Part model, mm, in its own coordinate system. Give positions to 0.01 mm unless a question says otherwise; leave off trailing zeros. Loops run counter-clockwise (first coordinate to the right, second up) from the corner with the lowest first, then second, coordinate; pieces in that order, holes last. Notation, with made-up numbers: M 74,55 L 103,55 A23 cw 103,69 Z; hole C 33,88.25 d4. An arc over 180 degrees is marked long. Put each result on its own line as item: value. Start each with the question number.
```python
from build123d import *

# Parameters (mm, degrees)
SKETCH1_W           = 271.5
SKETCH1_H           = 84
SKETCH1_R           = 1.5
BOSS_EXTRUDE1_DEPTH = 2
SKETCH2_R           = 1.5
SKETCH2_R_2         = 7.5
CUT_EXTRUDE1_DEPTH  = 10


with BuildPart() as part:
    # Sketch1 → Boss-Extrude1 (new body)
    with BuildSketch(Plane(origin=(0, 0, 0), x_dir=(1, 0, 0), z_dir=(0, 1, 0))):
        with Locations((135.75, 42)):
            Rectangle(SKETCH1_W, SKETCH1_H)
        with Locations(Location((4, 5.75, 0), (0, 0, 270))):
            Circle(SKETCH1_R, mode=Mode.SUBTRACT)
        with Locations(Location((4, 78.25, 0), (0, 0, 270))):
            Circle(SKETCH1_R, mode=Mode.SUBTRACT)
        with Locations(Location((267.5, 5.75, 0), (0, 0, 270))):
            Circle(SKETCH1_R, mode=Mode.SUBTRACT)
        with Locations(Location((267.5, 78.25, 0), (0, 0, 270))):
            Circle(SKETCH1_R, mode=Mode.SUBTRACT)
    extrude(amount=BOSS_EXTRUDE1_DEPTH)

    # Sketch2 → Cut-Extrude1 (cut)
    with BuildSketch(Plane(origin=(0, 2, 0), x_dir=(1, 0, 0), z_dir=(0, 1, 0))):
        with Locations(Location((15, 5.5, 0), (0, 0, 270))):
            Circle(SKETCH2_R)
        with Locations(Location((15, 40.5, 0), (0, 0, 270))):
            Circle(SKETCH2_R)
        with Locations(Location((15, 23, 0), (0, 0, 270))):
            Circle(SKETCH2_R_2)
        with Locations(Location((256.5, 23, 0), (0, 0, 90))):
            Circle(SKETCH2_R_2)
        with Locations(Location((256.5, 40.5, 0), (0, 0, 90))):
            Circle(SKETCH2_R)
        with Locations(Location((256.5, 5.5, 0), (0, 0, 90))):
            Circle(SKETCH2_R)
    extrude(amount=-CUT_EXTRUDE1_DEPTH, mode=Mode.SUBTRACT)


solid = part.part
```
1) Mould opens along Z. For faces 1 (the cylindrical face through (15.33, 1.014, -30.493)), 2 (the cylindrical face through (263.82, 1.01, -21.37)), 3 (the flat face through (134, 0, -43)) say: +Z half, -Z half, draft (parallel to the pull), parting line (faces both ways), or undercut.
2) Band-saw the part on A-A on z = -23. Give the cut face in (x, y).
3) Band-saw the part on B-B on y = 1.4. State how many separate pieces and enclosed holes the cut face has, then the cut area to 3 significant figures.
4) Pin check, flat tip, straight feed: pin 1 Ø9 at (x, z) = (15, -23) entering from +Y. Stop position of the tip, or through.
5) Wall check: L1, parallel to Z at x = 256.5, y = 1.3; L2, parallel to X at y = 0.4, z = -40.5; L3, parallel to Z at x = 267.5, y = 1.1. Give the ranges that are in metal, low to high.
Evaluation:
1. face 1: undercut
1. face 2: undercut
1. face 3: draft
2. outline: M 0,0 L 7.5,0 L 7.5,2 L 0,2 Z; M 22.5,0 L 249,0 L 249,2 L 22.5,2 Z; M 264,0 L 271.5,0 L 271.5,2 L 264,2 Z
3. separate pieces: 1
3. enclosed holes: 10
3. area: 22,400 mm2
4. pin 1: through
5. L1: -84 to -42, -39 to -30.5, -15.5 to -7, -4 to 0
5. L2: 0 to 13.5, 16.5 to 255, 258 to 271.5
5. L3: -84 to -79.75, -76.75 to -7.25, -4.25 to 0
